from build123d import *

# Parameters (mm, degrees)
BOSS_EXTRUDE1_DEPTH      = 3
SKETCH2_R                = 5
BOSS_EXTRUDE2_DEPTH      = 8
SKETCH3_R                = 5
BOSS_EXTRUDE3_DEPTH      = 92
BOSS_EXTRUDE6_DEPTH      = 9.2
BOSS_EXTRUDE7_REACH      = 190.339
BOSS_EXTRUDE7_END_RADIUS = 11
SKETCH8_W                = 3
SKETCH8_H                = 15
SKETCH9_R                = 2
CUT_EXTRUDE2_DEPTH       = 176.501823352
FILLET2_R                = 7.5


with BuildPart() as part:
    # Sketch1 → Boss-Extrude1 (new body)
    with BuildSketch(Plane.XY):
        with BuildLine():
            Line((0, 7.5), (150, 7.5))
            Line((150, 7.5), (150, -7.5))
            Line((150, -7.5), (0, -7.5))
            ThreePointArc((0, -7.5), (-7.5, 0), (0, 7.5))
        make_face()
    extrude(amount=BOSS_EXTRUDE1_DEPTH)

    # Sketch2 → Boss-Extrude2 (add)
    with BuildSketch(Plane.XY.offset(3)):
        Circle(SKETCH2_R)
    extrude(amount=BOSS_EXTRUDE2_DEPTH)

    # Sketch3 → Boss-Extrude3 (add)
    with BuildSketch(Plane.XY.offset(11)):
        Circle(SKETCH3_R)
    extrude(amount=BOSS_EXTRUDE3_DEPTH)

    # Sketch7 → Boss-Extrude6 (add)
    with BuildSketch(Plane.XY.offset(3)):
        with BuildLine():
            Line((136.95326153, 7.5), (132.009618943, 7.5))
            ThreePointArc((132.009618943, 7.5), (130, 0), (132.009618943, -7.5))
            Line((132.009618943, -7.5), (136.95326153, -7.5))
            ThreePointArc((136.95326153, -7.5), (134, 0), (136.95326153, 7.5))
        make_face()
    extrude(amount=BOSS_EXTRUDE6_DEPTH)

    # Boss-Extrude7: up to this cylinder (the profile starts inside it)
    boss_extrude7_end = Plane(origin=(145, 0, 10.7), z_dir=(0, 0, -1)) * Cylinder(BOSS_EXTRUDE7_END_RADIUS, 403.678, mode=Mode.PRIVATE)
    # Sketch8 → Boss-Extrude7 (add, up to the surface)
    with BuildSketch(Plane(origin=(150, 0, 0), x_dir=(0, 0, -1), z_dir=(1, 0, 0)), mode=Mode.PRIVATE) as boss_extrude7_sk1:
        with Locations((-10.7, 0)):
            Rectangle(SKETCH8_W, SKETCH8_H)
    boss_extrude7_tool1 = extrude(boss_extrude7_sk1.sketch, amount=-BOSS_EXTRUDE7_REACH, mode=Mode.PRIVATE) & boss_extrude7_end
    add(boss_extrude7_tool1.solids().sort_by_distance((150, 0, 10.7))[0])

    # Sketch9 → Cut-Extrude2 (cut, through all)
    with BuildSketch(Plane.XY.offset(12.2)):
        with Locations((142, 0)):
            Circle(SKETCH9_R)
    extrude(amount=-CUT_EXTRUDE2_DEPTH, mode=Mode.SUBTRACT)

    # Fillet2
    fillet2_edges = [part.edges().sort_by_distance(p)[0] for p in [
        (150, -7.5, 1.5),
        (150, -7.5, 10.7),
        (150, 7.5, 1.5),
        (150, 7.5, 10.7),
    ]]
    fillet(fillet2_edges, radius=FILLET2_R - 0.0001)  # a hair under: the kernel refuses the full size


solid = part.part
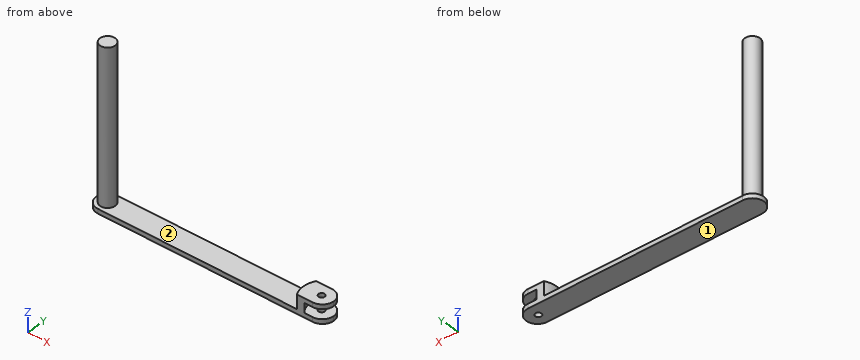
Here's how the part is built. I have some questions about the finished solid (model axes, mm). Face numbers are marked on the shaded views. Coordinates: 2 decimals unless noted, no trailing zeros. Order: outer loops, then holes, each group sorted by start corner. A loop starts at its lowest first (then second) coordinate and runs counter-clockwise, first axis right, second up. Notation, with made-up numbers: (-10.75, -40) - (36.25, -40) arc R17 ccw to (36.25, -14) - close; hole circle Ø11 at (46, 28). An arc over 180 degrees is marked (long way). Use CSV: the item, a comma, the result in double quotes. Start each with the question number.
1. Suppose I cut it at B-B on z = 54.5. List the corners of the cut face in (x, y) for me.
2. If we mould it in two halves opening along X, with no side actions, what happens to the marked faces 1 and 2? For each: +X half, -X half, draft (parallel to the pull), parting line (faces both ways), or undercut.
3. Suppose I cut it at A-A on x = 84.5. List the corners of the cut face in (y, z) for me.
4. Please list where these lines run through material, in increasing order: line 1 (Y direction, x = 142, z = 10); line 2 (Z direction, x = 139, y = 1.5); line 3 (Z direction, x = 34, y = -3.75). Write a range as from..to.
5. I'm going to push flat-ended pins straight in: pin 1 (7.5 mm diameter, centred on x = 141.5, y = 0.5, fed in from +Z); pin 2 (4 mm diameter, centred on x = 69, y = -1, fed in from +Z); pin 3 (2.5 mm diameter, centred on x = 142, y = 0, fed in from +Z) (3 decimals). Where does each tip first touch, or does it pass through?
Output:
1,outline,"circle Ø10 at (0, 0)"
2,face 1,"draft"
2,face 2,"undercut"
3,outline,"(-7.5, 0) - (7.5, 0) - (7.5, 3) - (-7.5, 3) - close"
4,line 1,"y = -7.5..-2, 2..7.5"
4,line 2,"z = 0..3, 9.2..12.2"
4,line 3,"z = 0..3"
5,pin 1,"stops at z = 12.2"
5,pin 2,"stops at z = 3"
5,pin 3,"passes through"
